Input: part model. Units: mm. Frame: model coordinates. Face numbers are marked on the shaded views. A direction names the side the tool comes from. Give positions to 0.01 mm unless a question says otherwise; leave off trailing zeros. Order: outer loops, then holes, each group sorted by start corner. A loop starts at its lowest first (then second) coordinate and runs counter-clockwise, first axis right, second up. Notation, with made-up numbers: (60.25, -21) -> (111.25, -21) arc R34 cw to (111.25, 11) -> close; hole circle Ø11 at (11, 54). An arc over 180 degrees is marked (long way). Use a Markdown table: item, result. Add a question column.
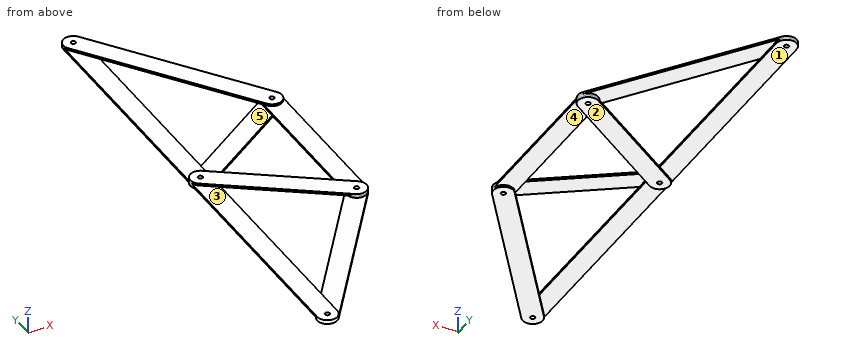
from build123d import *
from build123d.topology import SkipClean

# Parameters (mm, degrees)
CD_DEPTH                = 4.50787
BE_AE_DEPTH             = 4.50787
BOSS_EXTRUDE3_START     = -4.50787
BOSS_EXTRUDE3_DEPTH     = 4.50787
BOSS_EXTRUDE4_DEPTH     = 4.50787
BOSS_EXTRUDE5_START     = -4.50787
BOSS_EXTRUDE5_DEPTH     = 4.50787
BOSS_EXTRUDE7_DEPTH     = 4.50787
CUT_EXTRUDE1_DEPTH      = 784.294801
CUT_EXTRUDE1_DEPTH_BACK = 784.294801
SKETCH5_R               = 5.211191


with BuildPart() as part:
    # Sketch1 → CD (new body)
    with BuildSketch(Plane(origin=(0, 0, 0), x_dir=(0, 1, 0), z_dir=(0, 0, 1))):
        with BuildLine():
            Line((0, 22.539325), (354.92135, 22.539325))
            ThreePointArc((354.92135, 22.539325), (377.460675, 0), (354.92135, -22.539325))
            Line((354.92135, -22.539325), (0, -22.539325))
            ThreePointArc((0, -22.539325), (-22.539325, 0), (0, 22.539325))
        make_face()
    extrude(amount=CD_DEPTH)



with BuildPart() as body_2:
    # Sketch1<4> → BE & AE (new body)
    with BuildSketch(Plane(origin=(0, 0, 0), x_dir=(0, 1, 0), z_dir=(0, 0, 1))):
        with BuildLine():
            Line((177.460675, 277.460675), (-354.92135, 277.460675))
            ThreePointArc((-354.92135, 277.460675), (-377.460675, 254.92135), (-354.92135, 232.382025))
            Line((-354.92135, 232.382025), (177.460675, 232.382025))
            ThreePointArc((177.460675, 232.382025), (154.92135, 254.92135), (177.460675, 277.460675))
        make_face()
        with BuildLine():
            Line((709.8427, 277.460675), (177.460675, 277.460675))
            ThreePointArc((177.460675, 277.460675), (200, 254.92135), (177.460675, 232.382025))
            Line((177.460675, 232.382025), (709.8427, 232.382025))
            ThreePointArc((709.8427, 232.382025), (732.382025, 254.92135), (709.8427, 277.460675))
        make_face()
        with BuildLine():
            ThreePointArc((177.460675, 232.382025), (200, 254.92135), (177.460675, 277.460675))
            ThreePointArc((177.460675, 277.460675), (154.92135, 254.92135), (177.460675, 232.382025))
        make_face()
    extrude(amount=BE_AE_DEPTH)


with BuildPart() as part_1:
    add(part.part)

    add(body_2.part)  # Boss-Extrude3 merges body 2
    # Sketch1<5> → Boss-Extrude3 (add)
    with BuildSketch(Plane(origin=(0, 0, 0), x_dir=(0, 1, 0), z_dir=(0, 0, 1)).offset(BOSS_EXTRUDE3_START)):
        with BuildLine():
            Line((-341.772655, 273.227988), (13.148695, 18.306638))
            ThreePointArc((13.148695, 18.306638), (18.306638, -13.148695), (-13.148695, -18.306638))
            Line((-13.148695, -18.306638), (-368.070045, 236.614712))
            ThreePointArc((-368.070045, 236.614712), (-373.227988, 268.070045), (-341.772655, 273.227988))
        make_face()
    extrude(amount=BOSS_EXTRUDE3_DEPTH)

    # Sketch3 → Boss-Extrude4 (add)
    with BuildSketch(Plane.XY.offset(4.50787)):
        with BuildLine():
            Line((12.877475, 18.498427), (-242.043875, 195.959102))
            ThreePointArc((-242.043875, 195.959102), (-273.419777, 190.33815), (-267.798825, 158.962248))
            Line((-267.798825, 158.962248), (-12.877475, -18.498427))
            ThreePointArc((-12.877475, -18.498427), (18.498427, -12.877475), (12.877475, 18.498427))
        make_face()
    extrude(amount=BOSS_EXTRUDE4_DEPTH)

    # Sketch1<6> → Boss-Extrude5 (add)
    with BuildSketch(Plane(origin=(0, 0, 0), x_dir=(0, 1, 0), z_dir=(0, 0, 1)).offset(BOSS_EXTRUDE5_START)):
        with BuildLine():
            Line((195.959102, 267.798825), (373.419777, 12.877475))
            ThreePointArc((373.419777, 12.877475), (367.798825, -18.498427), (336.422923, -12.877475))
            Line((336.422923, -12.877475), (158.962248, 242.043875))
            ThreePointArc((158.962248, 242.043875), (164.5832, 273.419777), (195.959102, 267.798825))
        make_face()
    extrude(amount=BOSS_EXTRUDE5_DEPTH)

    # Sketch4 → Boss-Extrude7 (add)
    with SkipClean():  # the faces are left unmerged after this step: merging them gives an invalid solid
        with BuildSketch(Plane.XY.offset(4.50787)):
            with BuildLine():
                Line((-236.614712, 722.991395), (18.306638, 368.070045))
                ThreePointArc((18.306638, 368.070045), (13.148695, 336.614712), (-18.306638, 341.772655))
                Line((-18.306638, 341.772655), (-273.227988, 696.694005))
                ThreePointArc((-273.227988, 696.694005), (-268.070045, 728.149338), (-236.614712, 722.991395))
            make_face()
        extrude(amount=BOSS_EXTRUDE7_DEPTH)

    # Sketch5 → Cut-Extrude1 (cut, two sides: drawn at the far end of the back side and taken through both)
    with SkipClean():  # the faces are left unmerged after this step: merging them gives an invalid solid
        with BuildSketch(Plane.XY.offset(9.01574).offset(-CUT_EXTRUDE1_DEPTH_BACK)):
            Circle(SKETCH5_R)
            with Locations((-254.92135, 177.460675)):
                Circle(SKETCH5_R)
            with Locations((-254.92135, -354.92135)):
                Circle(SKETCH5_R)
            with Locations((0, 354.92135)):
                Circle(SKETCH5_R)
            with Locations((-254.92135, 709.8427)):
                Circle(SKETCH5_R)
        extrude(amount=CUT_EXTRUDE1_DEPTH + CUT_EXTRUDE1_DEPTH_BACK, mode=Mode.SUBTRACT)


solid = part_1.part
Q1. Section query A-A (y = -160). Return loops of the section in (x, z).
Q2. Ray query, line 1 (Y direction, x = 0, z = 1.5); line 2 (X direction, y = 336.5, z = 1.75); line 3 (Z direction, x = -223, y = 671). Return the intervals inside material, ascending.
Q3. Section query B-B (x = -220.5). Return loops of the section in (y, z).
Q4. Access query for the marked faces 1, 2 and 3. Directions: +Z, -Z, +X, -X, +Y, -Y. A direction counts if a zero-diameter tool reaches every point of the face in a straight line with its end or side. Return the directions, or none.
Q5. First-contact query: pin 1 (2 mm diameter, centred on y = -77.5, z = -0.5, fed in from +X); pin 2 (13.5 mm diameter, centred on x = -260, y = 439, fed in from -Z); pin 3 (5 mm diameter, centred on y = -114, z = 3, fed in from +X); pin 4 (16.5 mm diameter, centred on x = -254.92, y = 709.84, fed in from +Z). Flat tips, straight axial feed; report the tip coordinate or a pass-through.
Q6. Draft query along X for the marked faces 4 and 5. Return one class per face: +X half, -X half, draft (parallel to the pull), parting line (faces both ways), or undercut.
Solution:
| question | item | result |
|---|---|---|
| 1 | outline | (-277.46, 0) -> (-232.38, 0) -> (-232.38, 4.51) -> (-277.46, 4.51) -> close; (-142.67, -4.51) -> (-87.17, -4.51) -> (-87.17, 0) -> (-142.67, 0) -> close |
| 2 | line 1 | y = -22.54 to -5.21, 5.21 to 349.71, 360.13 to 377.46 |
| 2 | line 2 | x = -277.46 to -232.38, -22.54 to 22.54 |
| 2 | line 3 | z = 4.51 to 9.02 |
| 3 | outline | (-345.63, -4.51) -> (-268.36, -4.51) -> (-268.36, 0) -> (-345.63, 0) -> close; (126.04, 4.51) -> (180.96, 4.51) -> (180.96, 9.02) -> (126.04, 9.02) -> close; (173.96, -4.51) -> (228.89, -4.51) -> (228.89, 0) -> (173.96, 0) -> close; (623.28, 4.51) -> (700.56, 4.51) -> (700.56, 9.02) -> (623.28, 9.02) -> close |
| 4 | face 1 | -Z, -X, +Y |
| 4 | face 2 | -Z, +X, -X, +Y, -Y |
| 4 | face 3 | +Z, -X, -Y |
| 5 | pin 1 | stops at x = -27.2 |
| 5 | pin 2 | stops at z = 0 |
| 5 | pin 3 | stops at x = -232.38 |
| 5 | pin 4 | stops at z = 9.02 |
| 6 | face 4 | draft |
| 6 | face 5 | undercut |
